Check sheet for the modelled part. Datum: model origin and axes. Units: mm. Round coordinates to 2 decimals unless told otherwise and drop trailing zeros. Order: outer loops, then holes, each group sorted by start corner. A loop starts at its lowest first (then second) coordinate and runs counter-clockwise, first axis right, second up.
```python
from build123d import *

# Parameters (mm, degrees)
SALIENTE_EXTRUIR1_DEPTH = 3
REDONDEO1_R             = 0.5


with BuildPart() as part:
    # Croquis1 → Saliente-Extruir1 (new body)
    with BuildSketch(Plane.XY):
        with BuildLine():
            Line((0, 0), (82.2, 0))
            Line((82.2, 0), (82.2, 2.45))
            Line((82.2, 2.45), (2.95, 2.45))
            Line((2.95, 2.45), (2.95, 60))
            Line((2.95, 60), (0, 60))
            Line((0, 60), (0, 33.328427125))
            ThreePointArc((0, 33.328427125), (1, 30.5), (0, 27.671572875))
            Line((0, 27.671572875), (0, 0))
        make_face()
    extrude(amount=SALIENTE_EXTRUIR1_DEPTH)

    # Redondeo1
    redondeo1_edges = [part.edges().sort_by_distance(p)[0] for p in [
        (0, 60, 1.5),
        (82.2, 0, 1.5),
        (0, 0, 1.5),
    ]]
    fillet(redondeo1_edges, radius=REDONDEO1_R)


solid = part.part
```
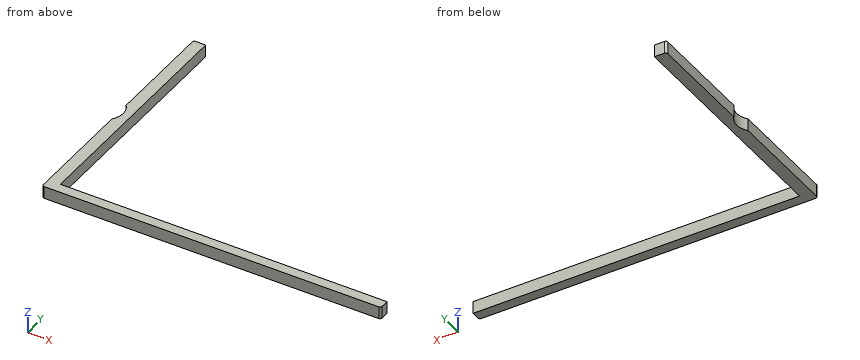
Item 1: Sectioned sample at B-B (x = 30.5). Record the cut outline in (y, z).
Answer:
outline: (0, 0) - (2.45, 0) - (2.45, 3) - (0, 3) - close
Item 2: Sectioned sample at A-A (z = 2). Record the cut outline in (x, y).
Answer:
outline: (0, 0.5) arc R0.5 ccw to (0.5, 0) - (81.7, 0) arc R0.5 ccw to (82.2, 0.5) - (82.2, 2.45) - (2.95, 2.45) - (2.95, 60) - (0.5, 60) arc R0.5 ccw to (0, 59.5) - (0, 33.33) arc R4.5 cw to (0, 27.67) - close
Item 3: Go/stop test with flat-tipped pins: P1, Ø1.5, axis at x = 23.5, z = 2, coming from the +Y side; P2, Ø1.5, axis at y = 19.5, z = 1.5, coming from the +X side. Record where each tip stops, or that it passes through.
Answer:
P1: stops at y = 2.45
P2: stops at x = 2.95
Item 4: Scan lines: line 1 along Y through (x, z) = (15, 1.95); line 2 along X through (y, z) = (36, 0.9). Record each from-to range of solid material in increasing order.
Answer:
line 1: y = 0 to 2.45
line 2: x = 0 to 2.95
Item 5: Sectioned sample at C-C (y = 47). Record the cut outline in (x, z).
Answer:
outline: (0, 0) - (2.95, 0) - (2.95, 3) - (0, 3) - close
